```python
from build123d import *

# Parameters (mm, degrees)
SKETCH_W        = 55
SKETCH_H        = 60
PAD_DEPTH       = 14
SKETCH001_R     = 7.6
POCKET_DEPTH    = 60.001
SKETCH002_R     = 1.75
POCKET001_DEPTH = 14.001
POCKET002_DEPTH = 12
SKETCH004_R     = 2.25
POCKET003_DEPTH = 14.001
SKETCH008_R     = 4.1
POCKET005_DEPTH = 20
SKETCH010_W     = 20
SKETCH010_H     = 25
POCKET006_DEPTH = 5
CHAMFER_SIZE    = 3
CHAMFER001_SIZE = 3


with BuildPart() as part:
    # Sketch → Pad (new body)
    with BuildSketch(Plane.XY):
        with Locations((17.5, 0)):
            Rectangle(SKETCH_W, SKETCH_H)
    extrude(amount=PAD_DEPTH)

    # Sketch001 → Pocket (cut, through all)
    with BuildSketch(Plane.XZ.offset(30)):
        with Locations((0, 14)):
            Circle(SKETCH001_R)
    extrude(amount=-POCKET_DEPTH, mode=Mode.SUBTRACT)

    # Sketch002 → Pocket001 (cut, through all)
    with BuildSketch(Plane(origin=(0, 0, 0), x_dir=(1, 0, 0), z_dir=(0, 0, -1))):
        with Locations((-6, 27)):
            Circle(SKETCH002_R)
        with Locations((36, 27)):
            Circle(SKETCH002_R)
        with Locations((-6, -27)):
            Circle(SKETCH002_R)
        with Locations((36, -27)):
            Circle(SKETCH002_R)
        with Locations((6, 27)):
            Circle(SKETCH002_R)
        with Locations((6, -27)):
            Circle(SKETCH002_R)
        with Locations((6, 0)):
            Circle(SKETCH002_R)
        with Locations((-6, 0)):
            Circle(SKETCH002_R)
        with Locations((36, -13)):
            Circle(SKETCH002_R)
        with Locations((36, 13)):
            Circle(SKETCH002_R)
    extrude(amount=-POCKET001_DEPTH, mode=Mode.SUBTRACT)

    # Sketch003 → Pocket002 (cut)
    with BuildSketch(Plane.XY.offset(14)):
        with BuildLine():
            Line((10, 35), (10, -35))
            Line((10, -35), (28, -35))
            Line((28, -35), (28, -14.916198))
            ThreePointArc((28, -14.916198), (30.841983, -12.965458), (32.599342, -10))
            Line((32.599342, -10), (52.599342, -10))
            Line((52.599342, -10), (52.599342, 10))
            Line((52.599342, 10), (32.599342, 10))
            ThreePointArc((32.599342, 10), (30.841983, 12.965458), (28, 14.916198))
            Line((28, 14.916198), (28, 35))
            Line((28, 35), (10, 35))
        make_face()
    extrude(amount=-POCKET002_DEPTH, mode=Mode.SUBTRACT)

    # Sketch004 → Pocket003 (cut, through all)
    with BuildSketch(Plane(origin=(0, 0, 0), x_dir=(1, 0, 0), z_dir=(0, 0, -1))):
        with Locations((25, 7.5)):
            Circle(SKETCH004_R)
        with Locations((25, -7.5)):
            Circle(SKETCH004_R)
    extrude(amount=-POCKET003_DEPTH, mode=Mode.SUBTRACT)

    # Sketch008 → Pocket005 (cut)
    with BuildSketch(Plane.YZ.offset(45)):
        with Locations((-20, 14)):
            Circle(SKETCH008_R)
        with Locations((20, 14)):
            Circle(SKETCH008_R)
    extrude(amount=-POCKET005_DEPTH, mode=Mode.SUBTRACT)

    # Sketch010 → Pocket006 (cut)
    with BuildSketch(Plane.YZ.offset(45)):
        with Locations((0, 6.5)):
            Rectangle(SKETCH010_W, SKETCH010_H)
    extrude(amount=-POCKET006_DEPTH, mode=Mode.SUBTRACT)

    # Chamfer
    chamfer_edges = [part.edges().sort_by_distance(p)[0] for p in [
        (45, -10, 8),
    ]]
    chamfer(chamfer_edges, length=CHAMFER_SIZE)

    # Chamfer001
    chamfer001_edges = [part.edges().sort_by_distance(p)[0] for p in [
        (45, 10, 8),
    ]]
    chamfer(chamfer001_edges, length=CHAMFER001_SIZE)


solid = part.part
```
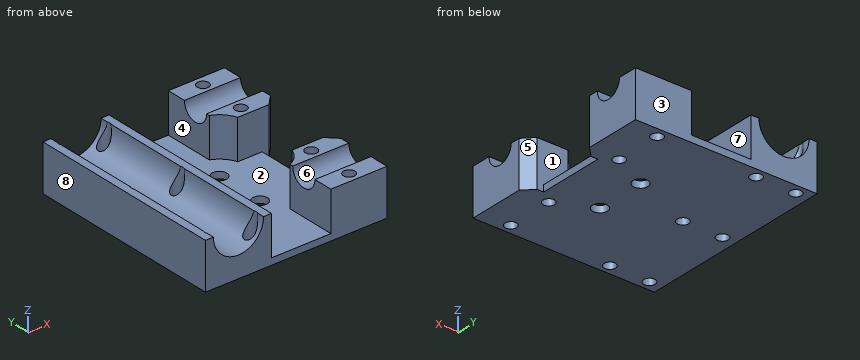
Can you work these out from the model? Positions are in its coordinate system, mm. Face numbers are marked on the shaded views. A direction names the side the tool comes from. Coordinates: 2 decimals unless noted, no trailing zeros. Write each loop counter-clockwise with the first axis right and the second up, starting at its lowest first coordinate (ties: lowest second). Pieces come first, ordered by that corner, then holes. Notation, with made-up numbers: M 44.5,18 L 52.5,18 A22 cw 52.5,25 Z; hole C 62.25,-4 d8. An arc over 180 degrees is marked long. Answer as CSV lines item,"result".
Item 1: Imagine slicing it at A-A on y = 7.5. List the corners of the cut face in (x, z) for me, plus the area to 3 significant figures.
Geometry results:
outline,"M -10,0 L 22.75,0 L 22.75,2 L 10,2 L 10,14 L 7.6,14 A7.6 cw -7.6,14 L -10,14 Z; M 27.25,0 L 40,0 L 40,2 L 27.25,2 Z"
area,"240 mm2"
Item 2: Imagine slicing it at D-D on x = 25. List the corners of the cut face in (y, z) for me.
Geometry results:
outline,"M -30,0 L -9.75,0 L -9.75,2 L -30,2 Z; M -5.25,0 L 5.25,0 L 5.25,2 L -5.25,2 Z; M 9.75,0 L 30,0 L 30,2 L 9.75,2 Z"
Item 3: Imagine slicing it at C-C on x = 36. List the corners of the cut face in (y, z) for me.
Geometry results:
outline,"M -30,0 L -28.75,0 L -28.75,14 L -30,14 Z; M -25.25,0 L -14.75,0 L -14.75,14 L -15.9,14 A4.1 cw -24.1,14 L -25.25,14 Z; M -11.25,0 L 11.25,0 L 11.25,14 L 10,14 L 10,2 L -10,2 L -10,14 L -11.25,14 Z; M 14.75,0 L 25.25,0 L 25.25,14 L 24.1,14 A4.1 cw 15.9,14 L 14.75,14 Z; M 28.75,0 L 30,0 L 30,14 L 28.75,14 Z"
Item 4: Imagine slicing it at B-B on z = 3.75. State how many separate pieces and enclosed holes the cut face has, plus the area to 3 significant figures.
Geometry results:
separate pieces,"3"
enclosed holes,"10"
area,"1,750 mm2"
Item 5: We'd pull the mould along X, two halves only. Please class the marked faces 5, 6, 7 and 8: +X half, -X half, draft (parallel to the pull), parting line (faces both ways), or undercut.
Geometry results:
face 5,"+X half"
face 6,"draft"
face 7,"undercut"
face 8,"-X half"
Item 6: On a 3-axis mill with a long thin cutter (end or side, diameter ignored), from which of +Z, -Z, +X, -X, +Y, -Y can I reach the whole of each face in a straight line? I mean the marked faces 1, 2, 3 and 4. Say none if no direction works.
Geometry results:
face 1,"+Z, +X"
face 2,"+Z"
face 3,"+Z, -Z, +X, -X, +Y"
face 4,"+Z, +Y, -Y"
Item 7: I'm going to push flat-ended pins straight in: P1, Ø5.5, axis at x = 36, y = -13, coming from the -Z side; P2, Ø1.6, axis at y = 3, z = 1, coming from the +X side; P3, Ø8, axis at x = -2, y = 3, coming from the +Z side. Where does each tip first touch, or does it pass through?
Geometry results:
P1,"stops at z = 0"
P2,"stops at x = 40"
P3,"stops at z = 9.34"
Item 8: Please list where these lines run through material, in increasing order: line 1 along X through (y, z) = (-27, 11); line 2 along Y through (x, z) = (36, 3.5); line 3 along X through (y, z) = (-27, 4.75).
Geometry results:
line 1,"x = -10 to -7.75, 7.75 to 10, 28 to 34.25, 37.75 to 45"
line 2,"y = -30 to -28.75, -25.25 to -14.75, -11.25 to -10, 10 to 11.25, 14.75 to 25.25, 28.75 to 30"
line 3,"x = -10 to -7.75, -4.25 to 4.25, 7.75 to 10, 28 to 34.25, 37.75 to 45"
